Work out the finished part from the listing and answer in its coordinate system (mm). A direction names the side the tool comes from. Coordinates: 2 decimals unless noted, no trailing zeros. Order: outer loops, then holes, each group sorted by start corner. A loop starts at its lowest first (then second) coordinate and runs counter-clockwise, first axis right, second up. Notation, with made-up numbers: M 58.25,-14 L 89.25,-14 A25 ccw 89.25,3 Z; hole C 28,-37.5 d4. An arc over 180 degrees is marked long. Use a Markdown table: item, result.
Autodesk Inventor part; units mm, degrees
ref_plane "YZ Plane" through (0, 0, 0) normal (1, 0, 0) x (0, 1, 0)
ref_plane "XZ Plane" through (0, 0, 0) normal (0, 1, 0) x (-1, 0, 0)
ref_plane "XY Plane" through (0, 0, 0) normal (0, 0, 1) x (1, 0, 0)
sketch "Sketch1" plane through (0, 0, 0) normal (0, 1, 0) x (-1, 0, 0)
  line L0 (122.8458, -138.2757) -> (56.882, -138.2757)
  line L1 (56.882, -138.2757) -> (56.882, -265.2757)
  line L2 (56.882, -265.2757) -> (122.8458, -265.2757)
  line L3 (122.8458, -265.2757) -> (122.8458, -138.2757)
  line L4 (110.1458, -173.9373) -> (69.582, -173.9373)
  line L5 (69.582, -173.9373) -> (69.582, -229.6141)
  line L6 (69.582, -229.6141) -> (110.1458, -229.6141)
  line L7 (110.1458, -229.6141) -> (110.1458, -173.9373)
  point P0 (0, 0)
  dimension "d1" = 127
  dimension "d4" = 55.6768
  dimension "d5" = 40.5638
  dimension "d6" = 12.7
  dimension "d7" = 35.6616
  dimension "d8" = 12.7
extrude "Extrusion1" add sketch "Sketch1" along normal blind 25.4 contours L3 L2 L1 L0 | L7 L6 L5 L4
shell "Shell1" thickness 2.54 removed faces 1 at (-56.882, 8.4667, -180.609)
sketch "Sketch3" plane through (0, 25.4, 0) normal (0, 1, 0) x (1, 0, 0)
  line L0 (-110.1458, 174.0389) -> (-69.582, 174.0389)
  line L1 (-69.582, 174.0389) -> (-69.582, 229.7157)
  line L2 (-69.582, 229.7157) -> (-110.1458, 229.7157)
  line L3 (-110.1458, 229.7157) -> (-110.1458, 174.0389)
  line L4 (-122.8458, 265.2757) -> (-122.8458, 138.2757)
  line L5 (-56.882, 265.2757) -> (-122.8458, 265.2757)
  point P0 (0, 0)
  dimension "d14" = 55.6768
  dimension "d15" = 40.5638
  dimension "d16" = 12.7
  dimension "d17" = 35.56
extrude "Extrusion2" cut sketch "Sketch3" against normal blind 12.7
sketch "Sketch4" plane through (0, 25.4, 0) normal (0, 1, 0) x (1, 0, 0)
  circle A0 centre (-91.0958, 156.2589) radius 6.35
  line L0 (-69.582, 174.0389) -> (-110.1458, 174.0389)
  line L1 (-122.8458, 265.2757) -> (-122.8458, 138.2757)
  line L2 (-122.8458, 138.2757) -> (-56.882, 138.2757)
  line L3 (-69.582, 229.7157) -> (-69.582, 174.0389)
  line L4 (-69.582, 174.0389) -> (-110.1458, 174.0389)
  line L5 (-110.1458, 174.0389) -> (-110.1458, 229.7157)
  line L6 (-110.1458, 229.7157) -> (-69.582, 229.7157)
  line L7 (-122.8458, 138.2757) -> (-56.882, 138.2757)
  line L8 (-56.882, 138.2757) -> (-56.882, 265.2757)
  line L9 (-56.882, 265.2757) -> (-122.8458, 265.2757)
  line L10 (-122.8458, 265.2757) -> (-122.8458, 138.2757)
  circle A1 centre (-91.0958, 247.4957) radius 6.35
  point P0 (0, 0)
  dimension "d20" = 12.7
  dimension "d21" = 17.78
  dimension "d22" = 31.75
  dimension "d23" = 12.7
  dimension "d24" = 17.78
  dimension "d25" = 31.75
hole "Hole1" at (-91.0958, 25.4, -156.2589) at (-91.0958, 25.4, -247.4957) direction (0, -1, 0) diameter 12.7 depth 12.7 tip angle 118
sketch "Sketch5" plane through (0, 0, 0) normal (0, -1, 0) x (1, 0, 0)
  line L0 (-122.8458, -265.2757) -> (-122.8458, -138.2757)
  line L1 (-122.8458, -138.2757) -> (-56.882, -138.2757)
  line L2 (-122.8458, -265.2757) -> (-122.8458, -138.2757)
  line L3 (-56.882, -265.2757) -> (-122.8458, -265.2757)
  line L4 (-56.882, -138.2757) -> (-56.882, -265.2757)
  line L5 (-96.1758, -206.8557) -> (-86.0158, -206.8557)
  line L6 (-86.0158, -206.8557) -> (-86.0158, -196.6957)
  line L7 (-86.0158, -196.6957) -> (-96.1758, -196.6957)
  line L8 (-96.1758, -196.6957) -> (-96.1758, -206.8557)
  point P0 (0, 0)
  dimension "d33" = 10.16
  dimension "d34" = 10.16
  dimension "d35" = 26.67
  dimension "d36" = 58.42
extrude "Extrusion3" cut sketch "Sketch5" against normal blind 12.7 contours L8 L7 L6 L5
sketch "Sketch6" plane through (-122.8458, 0, -265.2757) normal (-1, 0, 0) x (0, 0, 1)
  circle A0 centre (63.5, 12.7) radius 8.89
  line L0 (127, 0) -> (127, 25.4)
  line L1 (0, 25.4) -> (127, 25.4)
  line L2 (116.7244, 19.05) -> (91.3244, 19.05)
  line L3 (91.3244, 19.05) -> (91.3244, 6.35)
  line L4 (91.3244, 6.35) -> (116.7244, 6.35)
  line L5 (116.7244, 6.35) -> (116.7244, 19.05)
  line L6 (0, 0) -> (127, 0)
  point P0 (265.2757, 0)
  dimension "d39" = 17.78
  dimension "d40" = 63.5
  dimension "d41" = 12.7
  dimension "d49" = 12.7
  dimension "d50" = 25.4
  dimension "d51" = 6.35
hole "Hole2" at (-122.8458, 12.7, -201.7757) direction (1, 0, 0) diameter 17.78 depth 12.7 tip angle 118
extrude "Extrusion4" cut sketch "Sketch6" against normal blind 12.7 contours L5 L4 L3 L2
sketch "Sketch7" plane through (-56.882, 0, -265.2757) normal (0, 0, -1) x (-1, 0, 0)
  circle A0 centre (15.2497, 12.7) radius 2.54
  line L0 (0, 25.4) -> (65.9638, 25.4)
  point P0 (-56.882, 0)
  dimension "d54" = 5.08
  dimension "d55" = 12.7
hole "Hole3" at (-72.1317, 12.7, -265.2757) direction (0, 0, 1) diameter 5.08 depth 12.7 tip angle 118
fillet "Fillet1" radius 6.35 2 edges at (-122.8458, 12.7, -265.2757) (-122.8458, 12.7, -138.2757)
equation "\"d7\" = -0.5 * d4 + 0.5 * d1"
equation "\"d8\" = d6"
properties part number "prototype1_third_eye_not_blind"
1. Section B-B on x = -64.5 is taken. Determine the outline of the cut face in (y, z).
Answers below:
| item | result |
|---|---|
| outline | M 0,-265.28 L 25.4,-265.28 L 25.4,-138.28 L 0,-138.28 Z; hole M 2.54,-262.74 L 22.86,-262.74 L 22.86,-140.82 L 2.54,-140.82 Z |
2. For faces 1 (the face through (-89, 13, -140.816)), 2 (the face through (-69.582, 24, -201)), 3 (the face through (-91, 1, -196.696)), 4 (the face through (-122, 19.05, -161)), determine the directions among +Z, -Z, +X, -X, +Y, -Y from which every point of the face is accessible in a straight line to the end or side of a thin tool.
Answers below:
| item | result |
|---|---|
| face 1 | +X |
| face 2 | +Y |
| face 3 | +Y, -Y |
| face 4 | +X, -X |
3. Section D-D on x = -107 is taken. Determine the outline of the cut face in (y, z).
Answers below:
| item | result |
|---|---|
| outline | M 0,-265.28 L 25.4,-265.28 L 25.4,-229.72 L 22.86,-229.72 L 22.86,-262.74 L 2.54,-262.74 L 2.54,-140.82 L 22.86,-140.82 L 22.86,-174.04 L 25.4,-174.04 L 25.4,-138.28 L 0,-138.28 Z |
4. Flat-ended cylindrical pins translate along their axes: P1, Ø1.3, axis at x = -122, y = 10, coming from the +Z side; P2, Ø11.5, axis at x = -91.1, z = -247.5, coming from the +Y side; P3, Ø3, axis at x = -76.5, z = -152.5, coming from the -Y side; P4, Ø3, axis at x = -122, y = 15, coming from the -Z side. Find the tip coordinate at first contact, or state that the pin passes through.
Answers below:
| item | result |
|---|---|
| P1 | z = -140.53 |
| P2 | y = 2.54 |
| P3 | y = 0 |
| P4 | z = -263.85 |
5. Section A-A on z = -186 is taken. Determine the outline of the cut face in (x, y), then the cut area to 3 significant figures.
Answers below:
| item | result |
|---|---|
| outline | M -122.85,0 L -56.88,0 L -56.88,2.54 L -120.31,2.54 L -120.31,22.86 L -110.15,22.86 L -110.15,25.4 L -122.85,25.4 Z; M -69.58,22.86 L -56.88,22.86 L -56.88,25.4 L -69.58,25.4 Z |
| area | 284 mm² |
6. Find the intervals of material crossed by probe 1 along Y at (x, z) = (-69.5, -250.5); probe 2 along Z at (x, y) = (-99, 14); probe 3 along Z at (x, y) = (-121.25, 12.7), in increasing order.
Answers below:
| item | result |
|---|---|
| probe 1 | 0 to 2.54, 22.86 to 25.4 |
| probe 2 | -265.28 to -262.74, -140.82 to -138.28 |
| probe 3 | -263.14 to -210.67, -192.89 to -173.95, -148.55 to -140.42 |
7. Section C-C on y = 12.7 is taken. Determine the outline of the cut face in (x, z).
Answers below:
| item | result |
|---|---|
| outline | M -122.85,-258.93 A6.35 ccw -116.5,-265.28 L -74.67,-265.28 L -74.67,-262.74 L -120.31,-262.74 L -120.31,-210.67 L -122.85,-210.67 Z; M -122.85,-192.89 L -120.31,-192.89 L -120.31,-173.95 L -122.85,-173.95 Z; M -122.85,-148.55 L -120.31,-148.55 L -120.31,-140.82 L -56.88,-140.82 L -56.88,-138.28 L -116.5,-138.28 A6.35 ccw -122.85,-144.63 Z; M -69.59,-265.28 L -56.88,-265.28 L -56.88,-262.74 L -69.59,-262.74 Z |
8. For a pull along Y with two mould halves and no side action, classify faces 5 (the face through (-120.306, 22, -203)), 6 (the face through (-67, 25.4, -201)), 7 (the face through (-90, 24, -229.716)) as +Y half, -Y half, draft (parallel to the pull), parting line (faces both ways), or undercut.
Answers below:
| item | result |
|---|---|
| face 5 | undercut |
| face 6 | +Y half |
| face 7 | draft |
